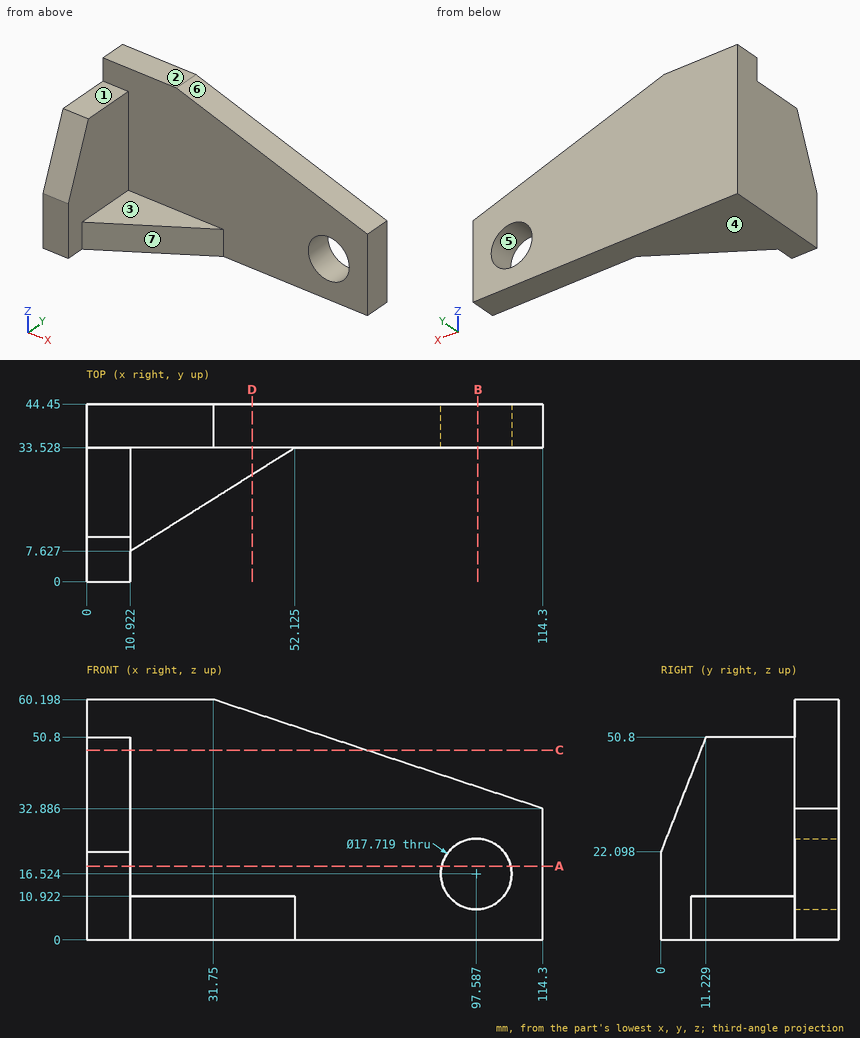
The drawing under review shows one solid part. Ordinate dimensions are in mm from its lowest x, y, z. A direction names the side the tool comes from. Round coordinates to 2 decimals unless told otherwise and drop trailing zeros. Loops run counter-clockwise (first coordinate to the right, second up) from the corner with the lowest first, then second, coordinate; pieces in that order, holes last. Notation, with made-up numbers: (6, 35) - (57, 35) arc R20 cw to (57, 61) - close; hole circle Ø9 at (-2, 8). An arc over 180 degrees is marked (long way). Use one line per item in the form item = value.
Item 1: Consider section A-A on z = 18.5. Write out the cut boundary in (x, y), then the cut area to 3 significant figures.
Answers:
outline = (0, 0) - (10.92, 0) - (10.92, 33.53) - (88.95, 33.53) - (88.95, 44.45) - (0, 44.45) - close; (106.22, 33.53) - (114.3, 33.53) - (114.3, 44.45) - (106.22, 44.45) - close
area = 1,430 mm^2
Item 2: Mouldability with a two-part tool opening along Z and no side actions: class the marked faces 4, 5, 6 and 7 as +Z half, -Z half, draft (parallel to the pull), parting line (faces both ways), or undercut.
Answers:
face_4 = -Z half
face_5 = undercut
face_6 = +Z half
face_7 = draft
Item 3: Clearance check with flat-ended pins moving along their axes: P1, Ø3.5, axis at x = 5, y = 23.5, coming from the +Z side; P2, Ø8, axis at x = 26.5, y = 21, coming from the +Z side; P3, Ø17, axis at y = 17, z = 22.5, coming from the +X side. State where each tip first meets the part, or that it passes through.
Answers:
P1 = 50.8
P2 = 10.92
P3 = 10.92
Item 4: Consider section D-D on x = 41.5. Write out the cut boundary in (y, z), then the cut area to 3 significant figures.
Answers:
outline = (26.85, 0) - (44.45, 0) - (44.45, 56.97) - (33.53, 56.97) - (33.53, 10.92) - (26.85, 10.92) - close
area = 695 mm^2
Item 5: Tool access review of the marked faces 1, 2 and 3: name each direction out of +Z, -Z, +X, -X, +Y, -Y from which nothing blocks a thin tool from reaching the whole face with its end or side.
Answers:
face_1 = +Z, +X, -X, -Y
face_2 = +Z, +X, -X, +Y, -Y
face_3 = +Z, +X, -Y
Item 6: For line 1 (Z direction, x = 13, y = 24); line 2 (Y direction, x = 53, z = 34), list the stretches that pass through material, from the lowest coordinate up.
Answers:
line_1 = 0 to 10.92
line_2 = 33.53 to 44.45
Item 7: Consider section C-C on z = 47.5. Write out the cut boundary in (x, y).
Answers:
outline = (0, 9.94) - (10.92, 9.94) - (10.92, 33.53) - (70.13, 33.53) - (70.13, 44.45) - (0, 44.45) - close
Item 8: Consider section B-B on x = 98. Write out the cut boundary in (y, z), then the cut area to 3 significant figures.
Answers:
outline = (33.53, 0) - (44.45, 0) - (44.45, 7.67) - (33.53, 7.67) - close; (33.53, 25.37) - (44.45, 25.37) - (44.45, 38.28) - (33.53, 38.28) - close
area = 225 mm^2
